from build123d import *

# Parameters (mm, degrees)
SKETCH_1_R          = 80
SKETCH_1_R_2        = 72
EXTRUDE_1_DEPTH     = 20
SKETCH_2_W          = 88.50052384
SKETCH_2_H          = 52
CUT_EXTRUDE_1_DEPTH = 20
SKETCH_3_W          = 5
SKETCH_3_H          = 8
EXTRUDE_2_DEPTH     = 20
FILLET_1_R          = 2
SKETCH_4_R          = 1.65
CUT_EXTRUDE_2_DEPTH = 20
SKETCH_5_R          = 3.05
CUT_EXTRUDE_3_DEPTH = 30
CUT_EXTRUDE_4_DEPTH = 50


with BuildPart() as part:
    # 草图1 → 凸台-拉伸1 (new body)
    with BuildSketch(Plane.XY):
        Circle(SKETCH_1_R)
        Circle(SKETCH_1_R_2, mode=Mode.SUBTRACT)
    extrude(amount=EXTRUDE_1_DEPTH)

    # 草图2 → 切除-拉伸1 (cut)
    with BuildSketch(Plane.XY.offset(20)):
        with Locations((-44.25026192, 54)):
            Rectangle(SKETCH_2_W, SKETCH_2_H)
    extrude(amount=-CUT_EXTRUDE_1_DEPTH, mode=Mode.SUBTRACT)

    # 草图3 → 凸台-拉伸2 (add)
    with BuildSketch(Plane.XY.offset(20)):
        with Locations((-2.5, 76)):
            Rectangle(SKETCH_3_W, SKETCH_3_H)
    extrude(amount=-EXTRUDE_2_DEPTH)

    # 圆角1
    fillet_1_edges = [part.edges().sort_by_distance(p)[0] for p in [
        (-66.332495807, 28, 10),
        (-74.939975981, 28, 10),
        (-5, 72, 10),
        (-5, 80, 10),
    ]]
    fillet(fillet_1_edges, radius=FILLET_1_R)

    # 草图4 → 切除-拉伸2 (cut)
    with BuildSketch(Plane.XY.offset(20)):
        with Locations((-76, 0)):
            Circle(SKETCH_4_R)
        with Locations((0, -76)):
            Circle(SKETCH_4_R)
        with Locations((76, 0)):
            Circle(SKETCH_4_R)
        with Locations((0, 76)):
            Circle(SKETCH_4_R)
    extrude(amount=-CUT_EXTRUDE_2_DEPTH, mode=Mode.SUBTRACT)

    # 草图5 → 切除-拉伸3 (cut)
    with BuildSketch(Plane.XY.offset(20)):
        with Locations((53.74011537, 53.74011537)):
            Circle(SKETCH_5_R)
        with Locations((53.74011537, -53.74011537)):
            Circle(SKETCH_5_R)
        with Locations((-53.74011537, -53.74011537)):
            Circle(SKETCH_5_R)
    extrude(amount=-CUT_EXTRUDE_3_DEPTH, mode=Mode.SUBTRACT)

    # 草图7 → 切除-拉伸4 (cut)
    with BuildSketch(Plane.XY.offset(20)):
        Polygon((6.869093861, -83.94322558), (-55.146771426, -64.405783947), (-66.191379441, -99.463645444), (-4.175514154, -119.001087078), align=None)
        Polygon((-8.271771426, 84.385124293), (53.744093861, 64.84768266), (64.788701876, 99.905544157), (2.772836589, 119.44298579), align=None)
    extrude(amount=-CUT_EXTRUDE_4_DEPTH, mode=Mode.SUBTRACT)


solid = part.part
Check sheet for the modelled part. Datum: model origin and axes. Units: mm. A direction names the side the tool comes from. Round coordinates to 2 decimals unless told otherwise and drop trailing zeros. Write each loop counter-clockwise with the first axis right and the second up, starting at its lowest first coordinate (ties: lowest second). Pieces come first, ordered by that corner, then holes. Notation, with made-up numbers: (-37.5, 46) -> (12.5, 46) arc R11 ccw to (12.5, 59) -> close; hole circle Ø11 at (-14, 8). An arc over 180 degrees is marked (long way). Answer as CSV lines item,"result". Start each with the question number.
1) Section check A-A on y = -59. Enter the section's corners in (x, z).
2) Section check D-D on y = 42. Enter the section's corners in (x, z), and give its area (3 significant figures).
3) Section check C-C on y = -25. Enter the section's corners in (x, z), and give its area (3 significant figures).
4) Material ranges on line 1 (X direction, y = -59.5, z = 4); line 2 (Y direction, x = -54.5, z = 3); line 3 (X direction, y = -63, z = 3.75), recorded low to high. Write a range as from..to.
5) Go/stop test with flat-tipped pins: P1, Ø1.5, axis at x = -1, z = 6, coming from the -Y side; P2, Ø2, axis at x = -46.5, z = 11, coming from the +Y side; P3, Ø2.5, axis at x = -76, y = 0, coming from the +Z side; P4, Ø1, axis at y = -7, z = 3.5, coming from the -X side. Record where each tip stops, or that it passes through.
6) Release check for a two-part mould opening along X. For faces 1 (the cylindrical face through (-75.39, -26.77, 9.86)), 2 (the cylindrical face through (51.49, 55.8, 10.14)), 3 (the flat face through (17, -71, 0)) record: pulls with the +X half, pulls with the -X half, needs draft (parallel to the pull), parting line crosses it, or undercut.
7) Section check B-B on z = 7. Enter the section's corners in (x, y), and give its area (3 significant figures).
8) Tool access check on faces 4 (the cylindrical face through (38.88, -60.6, 9.86)), 5 (the flat face through (-5, 76, 10)). Record the directions out of +Z, -Z, +X, -X, +Y, -Y that give a thin tool (end or side, any length) a straight path to the whole face; none if there is none.
Found:
1,outline,"(-54.03, 0) -> (-41.27, 0) -> (-41.27, 20) -> (-54.03, 20) -> close; (41.27, 0) -> (54.03, 0) -> (54.03, 20) -> (41.27, 20) -> close"
2,outline,"(58.48, 0) -> (68.09, 0) -> (68.09, 20) -> (58.48, 20) -> close"
2,area,"192 mm^2"
3,outline,"(-75.99, 0) -> (-67.52, 0) -> (-67.52, 20) -> (-75.99, 20) -> close; (67.52, 0) -> (75.99, 0) -> (75.99, 20) -> (67.52, 20) -> close"
3,area,"339 mm^2"
4,line 1,"x = -53.48..-40.54, 40.54..53.48"
4,line 2,"y = -58.56..-56.69, -50.79..-47.05"
4,line 3,"x = -49.31..-34.86, 34.86..49.31"
5,P1,"stops at y = -80"
5,P2,"stops at y = -54.11"
5,P3,"passes through"
5,P4,"stops at x = -79.74"
6,face 1,"pulls with the -X half"
6,face 2,"undercut"
6,face 3,"needs draft"
7,outline,"(-75.42, 26.67) arc R80 ccw to (-40.39, -69.05) -> (-6.48, -79.74) arc R80 ccw to (40.39, 69.05) -> (6.48, 79.74) arc R80 ccw to (0, 80) -> (-3, 80) arc R2 ccw to (-5, 78) -> (-5, 74) arc R2 ccw to (-3, 72) -> (0, 72) arc R72 cw (long way) to (-67.41, 25.3) arc R2 ccw to (-69.28, 28) -> (-73.54, 28) arc R2 ccw to start; hole circle Ø3.3 at (-76, 0); hole circle Ø6.1 at (-53.74, -53.74); hole circle Ø3.3 at (0, -76); hole circle Ø3.3 at (0, 76); hole circle Ø6.1 at (53.74, -53.74); hole circle Ø6.1 at (53.74, 53.74); hole circle Ø3.3 at (76, 0)"
7,area,"2,910 mm^2"
8,face 4,"+Z, -Z"
8,face 5,"+Z, -Z, -X, +Y"
